Check sheet for the modelled part. Datum: model origin and axes. Units: mm. Round coordinates to 2 decimals unless told otherwise and drop trailing zeros. Loops run counter-clockwise (first coordinate to the right, second up) from the corner with the lowest first, then second, coordinate; pieces in that order, holes last. Notation, with made-up numbers: (-30, 12.25) -> (-10, 12.25) arc R19 ccw to (-10, 43.25) -> close; hole circle Ø2 at (16, 20.5). An arc over 180 degrees is marked (long way). Use one line per item in the form item = value. Start each with the question number.
(1) Sectioned sample at C-C (z = 2). Record the cut outline in (x, y), and give its area (3 significant figures).
(2) Sectioned sample at A-A (z = -4). Record the cut outline in (x, y), and give its area (3 significant figures).
(3) Material ranges on probe 1 along Y at (x, z) = (-2.3, 1.25); probe 2 along Y at (x, z) = (1.1, 2); probe 3 along Z at (x, y) = (-1.25, 5.25), recorded low to high. Write a range as [from, to].
(4) Sectioned sample at D-D (y = 8). Record the cut outline in (x, z), and give its area (3 significant figures).
(5) Sectioned sample at B-B (x = 0). Record the cut outline in (y, z).
(6) Go/stop test with flat-tipped pins: pin 1 (1.3 mm diameter, centred on y = -0.5, z = -2.5, fed in from +X); pin 2 (3 mm diameter, centred on y = 3.5, z = 0.5, fed in from -X); pin 3 (3 mm diameter, centred on x = 0.5, y = 4, fed in from +Z). Record where each tip stops, or that it passes through.
from build123d import *

# Parameters (mm, degrees)
SKETCH2_W          = 0.4
SKETCH2_H          = 2.939387692
CUT_EXTRUDE1_DEPTH = 10.890399385
SKETCH3_W          = 0.5
SKETCH3_H          = 0.5


with BuildPart() as part:
    # Sketch1 → Revolve1 (revolve)
    with BuildSketch(Plane(origin=(0, 0, 0), x_dir=(1, 0, 0), z_dir=(0, 0, -1)), mode=Mode.PRIVATE) as revolve1_sk:
        with BuildLine():
            Line((0, 0), (0, -9))
            ThreePointArc((0, -9), (1.767766953, -8.267766953), (2.5, -6.5))
            Line((2.5, -6.5), (2.5, -1))
            Line((2.5, -1), (2.9, -1))
            Line((2.9, -1), (2.9, 0))
            Line((2.9, 0), (0, 0))
        make_face()
    revolve(revolve1_sk.sketch.rotate(Axis((0, 0, 0), (0, 1, 0)), 90), axis=Axis((0, 0, 0), (0, 1, 0)))

    # Sketch2 → Cut-Extrude1 (cut, through all)
    with BuildSketch(Plane(origin=(0, 0, 0), x_dir=(-1, 0, 0), z_dir=(0, -1, 0))):
        with Locations((-2.7, 0)):
            Rectangle(SKETCH2_W, SKETCH2_H)
    extrude(amount=-CUT_EXTRUDE1_DEPTH, mode=Mode.SUBTRACT)

    # Sweep1: sweep along a path in Sketch4
    with BuildLine(Plane(origin=(-1.27, 0, 0), x_dir=(0, 0, -1), z_dir=(1, 0, 0))) as sweep1_path:
        Line((0, 0), (0, -0.4))
        ThreePointArc((0, -0.4), (0.292893219, -1.107106781), (1, -1.4))
        Line((1, -1.4), (5, -1.4))
    # Sketch3 → Sweep1 (sweep)
    with BuildSketch(Plane(origin=(0, 0, 0), x_dir=(-1, 0, 0), z_dir=(0, -1, 0))):
        with Locations((-1.27, 0)):
            Rectangle(SKETCH3_W, SKETCH3_H)
        with Locations((1.27, 0)):
            Rectangle(SKETCH3_W, SKETCH3_H)
    sweep(path=sweep1_path.line)


solid = part.part
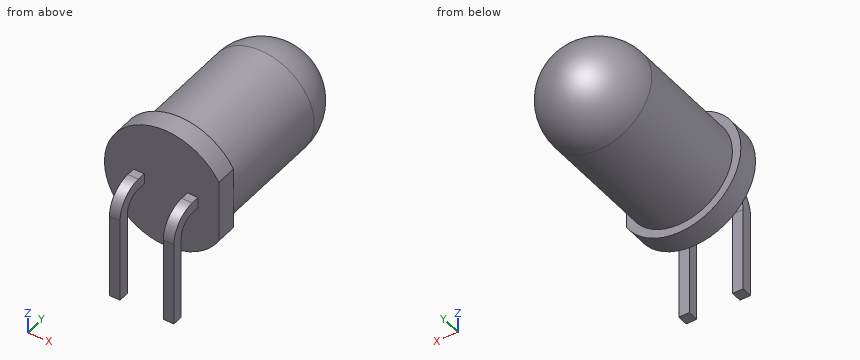
Checks:
q1.outline = (-2.1, 0) -> (2.1, 0) -> (2.1, 1) -> (1.5, 1) -> (1.5, 6.5) arc R1.5 ccw to (-1.5, 6.5) -> (-1.5, 1) -> (-2.1, 1) -> close
q1.area = 24.2 mm2
q2.outline = (-1.52, -1.65) -> (-1.02, -1.65) -> (-1.02, -1.15) -> (-1.52, -1.15) -> close; (1.02, -1.65) -> (1.52, -1.65) -> (1.52, -1.15) -> (1.02, -1.15) -> close
q2.area = 0.500 mm2
q3.probe_1 = [0, 1]
q3.probe_2 = [0, 7.52]
q3.probe_3 = [-2.17, 2.17]
q4.outline = circle Ø4 at (0, 0)
q4.area = 12.6 mm2
q5.outline = (0, -2.9) -> (1, -2.9) -> (1, -2.5) -> (6.5, -2.5) arc R2.5 ccw to (6.5, 2.5) -> (1, 2.5) -> (1, 2.9) -> (0, 2.9) -> close
q6.pin_1 = 2.02
q6.pin_2 = -2.5
q6.pin_3 = 2.5
